Geometry: final body of the model. Coordinates: model frame, mm. A direction names the side the tool comes from. Coordinates: 2 decimals unless noted, no trailing zeros. Order: outer loops, then holes, each group sorted by start corner. A loop starts at its lowest first (then second) coordinate and runs counter-clockwise, first axis right, second up. Notation, with made-up numbers: M -36.5,-10.5 L 4.5,-10.5 A29 ccw 4.5,12.5 Z; hole C 72.25,77.5 d8. An arc over 180 degrees is marked long. Use CSV: the item, a comma, the result in double quotes. Start each with the question number.
1. Section query C-C on x = 0. Return the cut outline in (y, z), and give its area (3 significant figures).
2. Section query B-B on y = 7.5. Return the cut outline in (x, z), and give its area (3 significant figures).
3. Section query A-A on z = 18. Return the cut outline in (x, y).
4. Section query D-D on z = 0. Return the cut outline in (x, y).
5. First-contact query: P1, Ø8, axis at y = 8.5, z = 14, coming from the -X side; P2, Ø4, axis at x = -14.5, y = 19.5, coming from the +Z side; P3, Ø9, axis at x = 18, y = 10, coming from the +Z side. Flat tips, straight axial feed; report the tip coordinate or a pass-through.
6. Set-up query: faces 1 (the flat face through (18, 6, 2)), 2 (the flat face through (-2, 6, 18)), 3 (the flat face through (18, 6, -2)). Return all of +Z, -Z, +X, -X, +Y, -Y with unobstructed straight access to the full face (end or side cutting, diameter ignored); none if empty.
7. Material intervals for line 1 (Y direction, x = -24.5, z = -18); line 2 (Z direction, x = 18, y = 3.5); line 3 (X direction, y = 21.5, z = 13.5), sorted ascending.
from build123d import *

# Parameters (mm, degrees)
SKETCH1_W           = 55
SKETCH1_H           = 55
BOSS_EXTRUDE1_DEPTH = 3
BOSS_EXTRUDE2_DEPTH = 2
CIRPATTERN1_COUNT   = 4
FILLET1_R           = 5


with BuildPart() as part:
    # Sketch1 → Boss-Extrude1 (new body)
    with BuildSketch(Plane(origin=(0, 0, 0), x_dir=(1, 0, 0), z_dir=(0, 1, 0))):
        Rectangle(SKETCH1_W, SKETCH1_H)
    extrude(amount=BOSS_EXTRUDE1_DEPTH)

    # Sketch2 → Revolve1 (revolve)
    with BuildSketch(Plane.XY):
        Polygon((0, 3), (0, 23), (15, 23), (15, 5.121320344), (17.121320344, 3), align=None)
    revolve(axis=Axis((0, 3, 0), (0, 1, 0)))

    # Sketch3 → Boss-Extrude2 (add, symmetric)
    with BuildSketch(Plane(origin=(0, 0, 0), x_dir=(0, 0, -1), z_dir=(1, 0, 0))):
        Polygon((10, 3), (10, 19), (26, 3), align=None)
    boss_extrude2 = extrude(amount=BOSS_EXTRUDE2_DEPTH, both=True)

    # CirPattern1: Boss-Extrude2 ×4 about axis
    cirpattern1_axis = Axis((0, 0, 0), (0, 1, 0))
    for i in range(1, CIRPATTERN1_COUNT):
        add(boss_extrude2.rotate(cirpattern1_axis, i * 360 / CIRPATTERN1_COUNT))

    # Fillet1
    fillet1_edges = [part.edges().sort_by_distance(p)[0] for p in [
        (-27.5, 1.5, -27.5),
        (27.5, 1.5, -27.5),
        (27.5, 1.5, 27.5),
        (-27.5, 1.5, 27.5),
    ]]
    fillet(fillet1_edges, radius=FILLET1_R)


solid = part.part
Results list:
1,outline,"M 0,-27.5 L 3,-27.5 L 3,-26 L 14,-15 L 23,-15 L 23,15 L 14,15 L 3,26 L 3,27.5 L 0,27.5 Z"
1,area,"886 mm²"
2,outline,"M -21.5,-2 L -14.87,-2 A15 ccw -2,-14.87 L -2,-21.5 L 2,-21.5 L 2,-14.87 A15 ccw 14.87,-2 L 21.5,-2 L 21.5,2 L 14.87,2 A15 ccw 2,14.87 L 2,21.5 L -2,21.5 L -2,14.87 A15 ccw -14.87,2 L -21.5,2 Z"
2,area,"812 mm²"
3,outline,"M -27.5,0 L 27.5,0 L 27.5,3 L 2,3 L 2,11 L -2,11 L -2,3 L -27.5,3 Z"
4,outline,"M -27.5,0 L 27.5,0 L 27.5,3 L 26,3 L 15,14 L 15,23 L -15,23 L -15,14 L -26,3 L -27.5,3 Z"
5,P1,"stops at x = -11.18"
5,P2,"stops at z = 8.29"
5,P3,"stops at z = 6.54"
6,face 1,"+Z, +X, +Y"
6,face 2,"+Z, -X, +Y"
6,face 3,"-Z, +X, +Y"
7,line 1,"y = 0 to 3"
7,line 2,"z = -2 to 2"
7,line 3,"x = -6.54 to 6.54"
